Build history of the part. All positions in model axes, mm. A direction names the side the tool comes from. Give positions to 0.01 mm unless a question says otherwise; leave off trailing zeros. Loops run counter-clockwise (first coordinate to the right, second up) from the corner with the lowest first, then second, coordinate; pieces in that order, holes last. Notation, with made-up numbers: M 86,39.5 L 103,39.5 A14 ccw 103,59.5 Z; hole C 66,40 d11. An arc over 180 degrees is marked long. Answer as a JSON object with one key per item and string values. Group by question number.
1. 3-axis set-ups, long thin cutter, end or side, ignore diameter. For faces 4 (the face through (47.06, 4.93, 5.366)), 5 (the face through (-46.273, 4.93, 9.625)), 6 (the face through (26.764, 4.93, -35.643)), 7 (the face through (30.61, 4.93, -36.15)): which of +Z, -Z, +X, -X, +Y, -Y reach the whole face in a straight line?
2. Drop flat-ended pins along their axis: pin 1 Ø2 at (y, z) = (8, 22.5) entering from -X; pin 2 Ø5 at (y, z) = (4.5, 15) entering from -X; pin 3 Ø1.5 at (y, z) = (6.5, 27.5) entering from -X. Give the stop position or say it passes through.
3. Mould opens along Z. For faces 1 (the face through (-10.4, 0, 10.4)), 2 (the face through (-39.526, 4.93, -25.914)), 3 (the face through (49.944, 4.93, -2.363)) say: released by +Z, released by -Z, zero draft, split by the parting line, or undercut.
4. Drill centre lines: line 1 along X through (y, z) = (7, 39.5); line 2 along X through (y, z) = (5.5, 34.5); line 3 along Z through (x, y) = (-9.5, 2.5). Where is each one in solid material? Low to high. Write a range as [from, to].
5. Slice it at A-A (x = 2.5). List the corners of the cut face in (y, z), then the cut area to 3 significant figures.
from build123d import *

# Parameters (mm, degrees)
CROQUIS1_R              = 50
SALIENTE_EXTRUIR1_DEPTH = 10
CROQUIS2_R              = 15
CORTAR_EXTRUIR1_DEPTH   = 10
CORTAR_EXTRUIR14_START  = -14
CORTAR_EXTRUIR14_DEPTH  = 14
MATRIZC1_COUNT          = 32


with BuildPart() as part:
    # Croquis1 → Saliente-Extruir1 (new body)
    with BuildSketch(Plane(origin=(0, 0, 0), x_dir=(1, 0, 0), z_dir=(0, 1, 0))):
        with Locations(Location((0, 0, 0), (0, 0, 270))):
            Circle(CROQUIS1_R)
    extrude(amount=SALIENTE_EXTRUIR1_DEPTH)

    # Croquis2 → Cortar-Extruir1 (cut)
    with BuildSketch(Plane(origin=(0, 10, 0), x_dir=(1, 0, 0), z_dir=(0, 1, 0))):
        with Locations(Location((0, 0.926579846, 0), (0, 0, 270))):
            Circle(CROQUIS2_R)
    extrude(amount=-CORTAR_EXTRUIR1_DEPTH, mode=Mode.SUBTRACT)

    # Croquis3 → Cortar-Extruir14 (cut)
    with BuildSketch(Plane(origin=(0, 10, 0), x_dir=(1, 0, 0), z_dir=(0, 1, 0)).offset(CORTAR_EXTRUIR14_START)):
        with BuildLine():
            Line((4.72393128, 44.406561165), (0.113748969, 44.606905854))
            Line((0.113748969, 44.606905854), (-0.954422894, 49.990889939))
            ThreePointArc((-0.954422894, 49.990889939), (2.523841382, 49.936261621), (5.989888947, 49.639915697))
            Line((5.989888947, 49.639915697), (4.72393128, 44.406561165))
        make_face()
    cortar_extruir14 = extrude(amount=CORTAR_EXTRUIR14_DEPTH, mode=Mode.SUBTRACT)

    # MatrizC1: Cortar-Extruir14 ×32 about axis
    matrizc1_axis = Axis((0, 0, 0), (0, 1, 0))
    for i in range(1, MATRIZC1_COUNT):
        add(cortar_extruir14.rotate(matrizc1_axis, i * 360 / MATRIZC1_COUNT), mode=Mode.SUBTRACT)


solid = part.part
Established:
{
 "1": {"face 4": "+X, +Y, -Y", "face 5": "-X, +Y, -Y", "face 6": "+Y, -Y", "face 7": "-Z, +Y, -Y"},
 "2": {"pin 1": "stops at x = -45.14", "pin 2": "stops at x = -48.41", "pin 3": "stops at x = -40.72"},
 "3": {"face 1": "zero draft", "face 2": "undercut", "face 3": "released by -Z"},
 "4": {"line 1": "x = [-25.9, -21.56], [-20.75, 20.82], [27.03, 30.66]", "line 2": "x = [-33.65, -28.82], [-28.32, 28.32], [35.76, 36.19]", "line 3": "z = [-45.97, -12.53], [10.68, 43.56]"},
 "5": {"outline": "M 0,-44.5 L 10,-44.5 L 10,-15.72 L 0,-15.72 Z; M 0,13.86 L 10,13.86 L 10,49.94 L 0,49.94 Z", "area": "649 mm^2"}
}
